CAD build for the part. Positions are in the model's coordinates, mm. Coordinates: 2 decimals unless noted, no trailing zeros. Loops run counter-clockwise (first coordinate to the right, second up) from the corner with the lowest first, then second, coordinate; pieces in that order, holes last. Notation, with made-up numbers: (64.5, 46) - (94.5, 46) arc R25 ccw to (94.5, 71) - close; hole circle Ø2 at (25, -1.75). An arc over 180 degrees is marked (long way). Put each result on its own line as item: value.
Autodesk Inventor part; units mm, degrees
ref_plane "YZ Plane" through (0, 0, 0) normal (1, 0, 0) x (0, 1, 0)
ref_plane "XZ Plane" through (0, 0, 0) normal (0, 1, 0) x (-1, 0, 0)
ref_plane "XY Plane" through (0, 0, 0) normal (0, 0, 1) x (1, 0, 0)
sketch "Náčrt1" plane through (0, 0, 0) normal (0, 0, 1) x (1, 0, 0)
  line L0 (-5.05, 0) -> (5.05, 0)
  line L1 (0, -1.329763) -> (0, 6.054961)
  line L2 (-9.941711, 0) -> (9.941711, 0)
  line L3 (-5.719696, 3.366789) -> (-1.776776, 5)
  line L4 (-1.776776, 5) -> (1.776776, 5)
  line L5 (1.776776, 5) -> (5.719696, 3.366789)
  arc A0 (-5.719696, 3.366789) -> (-5.05, 0) centre (-5.05, 1.75) ccw
  arc A1 (5.05, 0) -> (5.719696, 3.366789) centre (5.05, 1.75) ccw
  line L6 (6.565544, 0.875) -> (6.060363, 0)
  line L7 (6.060363, 0) -> (5.05, 0)
  arc A2 (5.05, 0) -> (6.565544, 0.875) centre (5.05, 1.75) ccw
  line L8 (-5.05, 0) -> (-6.060363, 0)
  line L9 (-6.060363, 0) -> (-6.565544, 0.875)
  arc A3 (-6.565544, 0.875) -> (-5.05, 0) centre (-5.05, 1.75) ccw
  point P0 (0, 0)
  dimension "d0" = 135
  dimension "d1" = 1.75
  dimension "d2" = 13.6
  dimension "d3" = 5
  dimension "d12" = 60
extrude "Vysunutí1" add sketch "Náčrt1" along normal blind 100
chamfer "Zkosení1" distance 0.5 angle 70 6 edges at (3.7482, 4.1834, 100) (6.7071, 2.3125, 100) (0, 0, 100) (-6.7071, 2.3125, 100) (-3.7482, 4.1834, 100) (0, 5, 100) measured on face at (0.5923, 1.6667, 100)
chamfer "Zkosení2" distance 0.5 angle 70 6 edges at (0, 0, 0) (6.7071, 2.3125, 0) (3.7482, 4.1834, 0) (-6.7071, 2.3125, 0) (-3.7482, 4.1834, 0) (0, 5, 0) measured on face at (0.5923, 1.6667, 0)
sketch "Náčrt2" plane through (-6.060363, 0, 98.626261) normal (0, -1, 0) x (1, 0, 0)
  line L0 (6.060363, -118.626261) -> (6.060363, 21.373739)
  line L1 (-3.459637, -98.626261) -> (15.580363, -98.626261)
  line L2 (12.120726, -97.252523) -> (0, -97.252523)
  line L3 (12.120726, -97.252523) -> (12.120726, 0)
  line L4 (0, 0) -> (12.120726, 0)
  line L5 (0, -97.252523) -> (0, 0)
  line L6 (7.435363, -6.126261) -> (4.685363, -6.126261)
  line L7 (4.685363, -6.126261) -> (4.685363, -91.126261)
  line L8 (4.685363, -91.126261) -> (7.435363, -91.126261)
  line L9 (7.435363, -91.126261) -> (7.435363, -6.126261)
  line L10 (11.832051, 1.373739) -> (0.288675, 1.373739)
  point P0 (6.060363, -98.626261)
  dimension "d13" = 2.75
  dimension "d14" = 7.5
  dimension "d15" = 7.5
extrude "Vysunutí2" cut sketch "Náčrt2" against normal blind 2.5 contours L8 L7 L6 L0 | L0 L6 L9 L8
equation "\"d9\" = d6"
equation "\"d11\" = d8"
equation "\"d15\" = d14"
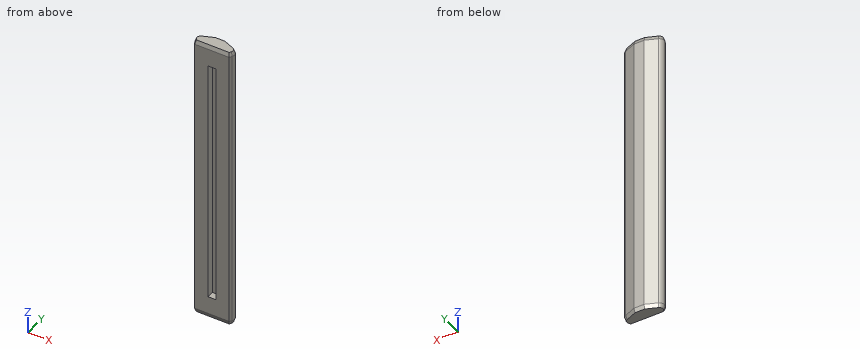
Q1. Wall check: L1, parallel to Z at x = 0.75, y = 1.25; L2, parallel to X at y = 0.45, z = 28 (3 decimals); L3, parallel to Y at x = 5.75, z = 92. Give the ranges that are in metal, low to high. Write a range as from..to.
Determined:
L1: 0..7.5, 92.5..100
L2: -6.32..-1.375, 1.375..6.32
L3: 0..3.35
Q2. Slice it at B-B, the plane z = 60. Give the cut face in (x, y) (3 decimals), then the cut area to 3 significant figures.
Determined:
outline: (-6.566, 0.875) - (-6.06, 0) - (-1.375, 0) - (-1.375, 2.5) - (1.375, 2.5) - (1.375, 0) - (6.06, 0) - (6.566, 0.875) arc R1.75 ccw to (5.72, 3.367) - (1.777, 5) - (-1.777, 5) - (-5.72, 3.367) arc R1.75 ccw to start
area: 49.2 mm2
Q3. Slice it at C-C, the plane x = -4.5. Give the cut face in (y, z), then the cut area to 3 significant figures.
Determined:
outline: (0, 1.37) - (0.5, 0) - (3.33, 0) - (3.87, 1.37) - (3.87, 98.63) - (3.33, 100) - (0.5, 100) - (0, 98.63) - close
area: 386 mm2
Q4. Slice it at D-D, the plane x = 4. Give the cut face in (y, z).
Determined:
outline: (0, 1.37) - (0.5, 0) - (3.54, 0) - (4.08, 1.37) - (4.08, 98.63) - (3.54, 100) - (0.5, 100) - (0, 98.63) - close
Q5. Pin check, flat tips, straight feed: pin 1 Ø6 at (x, z) = (3.5, 82) entering from +Y; pin 2 Ø1 at (y, z) = (3.5, 71.5) entering from +X; pin 3 Ø1.2 at (y, z) = (1, 30.5) entering from -X; pin 4 Ø1.2 at (y, z) = (1, 53) entering from +X. Stop position of each tip, or through.
Determined:
pin 1: y = 5
pin 2: x = 6.27
pin 3: x = -6.79
pin 4: x = 6.79
Q6. Slice it at A-A, the plane x = 0. Give the cut face in (y, z), then the cut area to 3 significant figures.
Determined:
outline: (0, 1.37) - (0.5, 0) - (4.5, 0) - (5, 1.37) - (5, 98.63) - (4.5, 100) - (0.5, 100) - (0, 98.63) - (0, 92.5) - (2.5, 92.5) - (2.5, 7.5) - (0, 7.5) - close
area: 286 mm2
